from build123d import *

# Parameters (mm, degrees)
BOSS_EXTRUDE1_DEPTH                       = 12.7
BOSS_EXTRUDE1_DEPTH_BACK                  = 12.7
CUT_EXTRUDE1_DEPTH                        = 83.589067678
CUT_EXTRUDE1_DEPTH_BACK                   = 83.589067678
SKETCH5_R                                 = 3.302
BOSS_EXTRUDE_START                        = -12.7
SKETCH10_W                                = 12.7
SKETCH10_H                                = 38.1
BOSS_EXTRUDE_ARM_FB_WIDTH_DEPTH           = 44.45
BOSS_EXTRUDE_ARM_CHASSIS_FB_DEPTH         = 95.25
SKETCH15_W                                = 55.88
SKETCH15_H                                = 38.1
BOSS_EXTRUDE_ARM_CHASSIS_LR_DEPTH         = 50.8
SKETCH16_R                                = 12.7635
CUT_EXTRUDE_CHASSIS_FB_DEPTH              = 128.199614864
SKETCH17_R                                = 12.7635
SKETCH17_W                                = 12.7635
SKETCH17_H                                = 38.1
CUT_EXTRUDE_CHASSIS_LR_DEPTH              = 128.199614864
CUT_EXTRUDE_START                         = -22.107857563
CUT_EXTRUDE_CHASSIS_JOINT_CLEARANCE_DEPTH = 43.685920391
SKETCH19_W                                = 25.4
SKETCH19_H                                = 5.08
BOSS_EXTRUDE_FB_CLAMP_TOP_DEPTH           = 7.62
BOSS_EXTRUDE_START_2                      = -38.1
SKETCH19_3_W                              = 25.4
SKETCH19_3_H                              = 5.08
BOSS_EXTRUDE_FB_CLAMP_BOTTOM_DEPTH        = 7.62
SKETCH20_W                                = 5.08
SKETCH20_H                                = 25.4
BOSS_EXTRUDE_LR_CLAMP_TOP_DEPTH           = 7.62
SKETCH20_3_W                              = 5.08
SKETCH20_3_H                              = 25.4
BOSS_EXTRUDE_LR_CLAMP_BOTTOM_DEPTH        = 7.62
CHAMFER1_SIZE                             = 0.508
CHAMFER2_SIZE                             = 30.48
CHAMFER7_SIZE                             = 5.08
SKETCH26_FB_CLAMP_HOLES_R                 = 1.625000052
CUT_EXTRUDE7_FB_HOLES_DEPTH               = 136.265877047
SKETCH23_LR_CLAMP_HOLES_R                 = 1.625000052
CUT_EXTRUDE8_FB_HOLES_DEPTH               = 114.46180152
CHAMFER8_SIZE                             = 0.508


# Read off the part's stored shape, not the designer's step: Cut-Extrude Chassis Joint Clearance
with BuildPart() as part:
    # Sketch3 → Boss-Extrude1 (new, two sides: drawn at the far end of the back side and taken through both)
    with BuildSketch(Plane(origin=(0, 0, 0), x_dir=(1, 0, 0), z_dir=(0, 1, 0)).offset(-BOSS_EXTRUDE1_DEPTH_BACK)):
        with BuildLine():
            Line((8.001, 0), (10.541, 0))
            ThreePointArc((10.541, 0), (8.89018923, 5.663675172), (4.454819097, 9.553390383))
            Line((4.454819097, 9.553390383), (-5.969, 14.414097055))
            Line((-5.969, 14.414097055), (-5.969, 40.894))
            Line((-5.969, 40.894), (-18.669, 40.894))
            Line((-18.669, 40.894), (-18.669, -76.2))
            Line((-18.669, -76.2), (-5.969, -76.2))
            Line((-5.969, -76.2), (-5.969, -5.327948949))
            ThreePointArc((-5.969, -5.327948949), (-2.851142929, 7.475759828), (8.001, 0))
        make_face()
    extrude(amount=BOSS_EXTRUDE1_DEPTH + BOSS_EXTRUDE1_DEPTH_BACK)

    # Sketch5 → Cut-Extrude1 (cut, two sides: drawn at the far end of the back side and taken through both)
    with BuildSketch(Plane.ZY.offset(18.669).offset(-CUT_EXTRUDE1_DEPTH_BACK)):
        with Locations((-21.844, 0)):
            Circle(SKETCH5_R)
        with Locations((21.844, 0)):
            Circle(SKETCH5_R)
    extrude(amount=CUT_EXTRUDE1_DEPTH + CUT_EXTRUDE1_DEPTH_BACK, mode=Mode.SUBTRACT)

    # Sketch10 → Boss-Extrude Arm FB Width (add)
    with BuildSketch(Plane.XZ.offset(12.7).offset(BOSS_EXTRUDE_START)):
        with Locations((-12.319, 57.15)):
            Rectangle(SKETCH10_W, SKETCH10_H)
    extrude(amount=BOSS_EXTRUDE_ARM_FB_WIDTH_DEPTH)

    # Sketch12 → Boss-Extrude Arm Chassis FB (add)
    with BuildSketch(Plane(origin=(-5.969, 0, 0), x_dir=(0, 0, -1), z_dir=(1, 0, 0))):
        Polygon((-38.1, 0), (-76.2, 0), (-76.2, -44.45), (-38.1, -44.45), (-38.1, -12.7), align=None)
    extrude(amount=BOSS_EXTRUDE_ARM_CHASSIS_FB_DEPTH)

    # Sketch15 → Boss-Extrude Arm Chassis LR (add)
    with BuildSketch(Plane(origin=(0, 0, 0), x_dir=(1, 0, 0), z_dir=(0, 1, 0))):
        with Locations((9.271, -57.15)):
            Rectangle(SKETCH15_W, SKETCH15_H)
    extrude(amount=BOSS_EXTRUDE_ARM_CHASSIS_LR_DEPTH)

    # Sketch16 → Cut-Extrude Chassis FB (cut, through all)
    with BuildSketch(Plane(origin=(32.122028853, -6.645348837, 57.15), x_dir=(0, 0, 1), z_dir=(-1, 0, 0))):
        Circle(SKETCH16_R)
        with BuildLine():
            Line((-19.05, 0), (-12.7635, 0))
            ThreePointArc((-12.7635, 0), (-9.025157412, 9.025157392), (-2.9e-08, 12.7635))
            Line((-2.9e-08, 12.7635), (-19.05, 12.7635))
            Line((-19.05, 12.7635), (-19.05, 0))
        make_face()
        with BuildLine():
            ThreePointArc((-2.9e-08, 12.7635), (9.025157392, 9.025157412), (12.7635, 0))
            Line((12.7635, 0), (19.05, 0))
            Line((19.05, 0), (19.05, 12.7635))
            Line((19.05, 12.7635), (-2.9e-08, 12.7635))
        make_face()
    extrude(amount=-CUT_EXTRUDE_CHASSIS_FB_DEPTH, mode=Mode.SUBTRACT)

    # Sketch17 → Cut-Extrude Chassis LR (cut, through all)
    with BuildSketch(Plane(origin=(32.122028853, -6.645348837, 57.15), x_dir=(1, 0, 0), z_dir=(0, 1, 0))):
        Circle(SKETCH17_R)
        with Locations((6.38175, 0)):
            Rectangle(SKETCH17_W, SKETCH17_H)
    extrude(amount=CUT_EXTRUDE_CHASSIS_LR_DEPTH, mode=Mode.SUBTRACT)

    # Cut-Extrude Chassis Joint Clearance outl → Cut-Extrude Chassis Joint Clearance (cut)
    with BuildSketch(Plane(origin=(0, 1.051977093, 58.045037899), x_dir=(1, 0, 0), z_dir=(0, -0.11550085817456393, 0.9933073803012538)).offset(CUT_EXTRUDE_START)):
        with BuildLine():
            Line((65.60424969, 4.087995405), (49.027279167, 4.087995405))
            ThreePointArc((49.027279167, 4.087995405), (41.651365859, 10.55649777), (32.122028853, 12.8883117))
            Line((32.122028853, 12.8883117), (32.122028853, 17.444547275))
            Line((32.122028853, 17.444547275), (20.284845148, 9.156062014))
            ThreePointArc((20.284845148, 9.156062014), (17.529112657, -22.342104497), (49.027279167, -19.586372005))
            Line((49.027279167, -19.586372005), (65.60424969, 4.087995405))
        make_face()
    extrude(amount=CUT_EXTRUDE_CHASSIS_JOINT_CLEARANCE_DEPTH, mode=Mode.SUBTRACT)

    # Sketch19 → Boss-Extrude FB Clamp Top (add)
    with BuildSketch(Plane.XY.offset(76.2)):
        with Locations((76.581, -9.185348837)):
            Rectangle(SKETCH19_W, SKETCH19_H)
    extrude(amount=BOSS_EXTRUDE_FB_CLAMP_TOP_DEPTH)

    # Sketch19<3> → Boss-Extrude FB Clamp Bottom (add)
    with BuildSketch(Plane.XY.offset(76.2).offset(BOSS_EXTRUDE_START_2)):
        with Locations((76.581, -9.185348837)):
            Rectangle(SKETCH19_3_W, SKETCH19_3_H)
    extrude(amount=-BOSS_EXTRUDE_FB_CLAMP_BOTTOM_DEPTH)

    # Sketch20 → Boss-Extrude LR Clamp Top (add)
    with BuildSketch(Plane.XY.offset(76.2)):
        with Locations((29.582028853, 38.1)):
            Rectangle(SKETCH20_W, SKETCH20_H)
    extrude(amount=BOSS_EXTRUDE_LR_CLAMP_TOP_DEPTH)

    # Sketch20<3> → Boss-Extrude LR Clamp Bottom (add)
    with BuildSketch(Plane.XY.offset(76.2).offset(BOSS_EXTRUDE_START_2)):
        with Locations((29.582028853, 38.1)):
            Rectangle(SKETCH20_3_W, SKETCH20_3_H)
    extrude(amount=-BOSS_EXTRUDE_LR_CLAMP_BOTTOM_DEPTH)

    # Chamfer1
    chamfer1_edges = [part.edges().sort_by_distance(p)[0] for p in [
        (76.581, -11.725348837, 76.2),
        (76.581, -11.725348837, 38.1),
    ]]
    chamfer(chamfer1_edges, length=CHAMFER1_SIZE)

    # Chamfer2
    chamfer2_edges = [part.edges().sort_by_distance(p)[0] for p in [
        (-18.669, 50.8, 57.15),
    ]]
    chamfer(chamfer2_edges, length=CHAMFER2_SIZE)

    # Chamfer7
    chamfer7_edges = [part.edges().sort_by_distance(p)[0] for p in [
        (-12.319, 12.7, 38.1),
        (-12.319, -12.7, 38.1),
    ]]
    chamfer(chamfer7_edges, length=CHAMFER7_SIZE)

    # Sketch26 FB Clamp Holes → Cut-Extrude7 FB Holes (cut, through all)
    with BuildSketch(Plane(origin=(0, -6.645348837, 0), x_dir=(1, 0, 0), z_dir=(0, 1, 0))):
        with Locations((70.281000154, -80.01)):
            Circle(SKETCH26_FB_CLAMP_HOLES_R)
        with BuildLine():
            Line((72.264758924, -80.01), (71.612122269, -79.077938261))
            ThreePointArc((71.612122269, -79.077938261), (71.830790249, -79.52135306), (71.906000206, -80.01))
            ThreePointArc((71.906000206, -80.01), (71.830790249, -80.49864694), (71.612122269, -80.942061739))
            Line((71.612122269, -80.942061739), (72.264758924, -80.01))
        make_face()
        with BuildLine():
            Line((84.2647588, -80.01), (83.612122145, -79.077938261))
            ThreePointArc((83.612122145, -79.077938261), (83.830790125, -79.52135306), (83.906000082, -80.01))
            ThreePointArc((83.906000082, -80.01), (83.830790125, -80.49864694), (83.612122145, -80.942061739))
            Line((83.612122145, -80.942061739), (84.2647588, -80.01))
        make_face()
        with Locations((82.28100003, -80.01)):
            Circle(SKETCH26_FB_CLAMP_HOLES_R)
        with BuildLine():
            Line((84.2647588, -34.29), (83.612122145, -33.357938261))
            ThreePointArc((83.612122145, -33.357938261), (83.830790125, -33.80135306), (83.906000082, -34.29))
            ThreePointArc((83.906000082, -34.29), (83.830790125, -34.77864694), (83.612122145, -35.222061739))
            Line((83.612122145, -35.222061739), (84.2647588, -34.29))
        make_face()
        with Locations((82.28100003, -34.29)):
            Circle(SKETCH26_FB_CLAMP_HOLES_R)
        with BuildLine():
            Line((72.264758924, -34.29), (71.612122269, -33.357938261))
            ThreePointArc((71.612122269, -33.357938261), (71.830790249, -33.80135306), (71.906000206, -34.29))
            ThreePointArc((71.906000206, -34.29), (71.830790249, -34.77864694), (71.612122269, -35.222061739))
            Line((71.612122269, -35.222061739), (72.264758924, -34.29))
        make_face()
        with Locations((70.281000154, -34.29)):
            Circle(SKETCH26_FB_CLAMP_HOLES_R)
    extrude(amount=-CUT_EXTRUDE7_FB_HOLES_DEPTH, mode=Mode.SUBTRACT)

    # Sketch23 LR Clamp Holes → Cut-Extrude8 FB Holes (cut, through all)
    with BuildSketch(Plane(origin=(32.122028853, 0, 0), x_dir=(0, 0, -1), z_dir=(1, 0, 0))):
        with Locations((-80.01, 43.80000003)):
            Circle(SKETCH23_LR_CLAMP_HOLES_R)
        with Locations((-80.01, 31.800000154)):
            Circle(SKETCH23_LR_CLAMP_HOLES_R)
        with Locations(Location((-34.29, 31.800000154, 0), (0, 0, 90))):
            Circle(SKETCH23_LR_CLAMP_HOLES_R)
        with Locations(Location((-34.29, 43.80000003, 0), (0, 0, 90))):
            Circle(SKETCH23_LR_CLAMP_HOLES_R)
    extrude(amount=-CUT_EXTRUDE8_FB_HOLES_DEPTH, mode=Mode.SUBTRACT)

    # Chamfer8
    chamfer8_edges = [part.edges().sort_by_distance(p)[0] for p in [
        (27.042028853, 38.1, 76.2),
        (27.042028853, 38.1, 38.1),
    ]]
    chamfer(chamfer8_edges, length=CHAMFER8_SIZE)


solid = part.part
Verification items for the finished model (mm, model axes). A direction names the side the tool comes from. Coordinates: 2 decimals unless noted, no trailing zeros. Loops run counter-clockwise (first coordinate to the right, second up) from the corner with the lowest first, then second, coordinate; pieces in that order, holes last. Notation, with made-up numbers: (44.5, -9.75) -> (96.5, -9.75) arc R19 cw to (96.5, 0.25) -> close; hole circle Ø10 at (55, 14). An arc over 180 degrees is marked (long way). Answer as a JSON object with one key per item and string values. Group by question number.
Item 1: Sectioned sample at B-B on y = 43.8. State how many separate pieces and enclosed holes the cut face has, plus the area to 3 significant figures.
Item 2: Mould release check, pull along X, two halves, no side actions. Record for faces 1 (the cylindrical face through (80.657, -9.15, 34.232)), 2 (the flat face through (27.042, 38, 80)), 3 (the flat face through (17, 50.8, 58)): +X half, -X half, draft (parallel to the pull), parting line (faces both ways), or undercut.
Item 3: Tool access check on faces 4 (the flat face through (27.042, 38, 34)), 5 (the flat face through (-11, 12.7, -4)), 6 (the flat face through (74, -6.645, 77)), 7 (the flat face through (63.881, -9, 34)). Record the directions out of +Z, -Z, +X, -X, +Y, -Y that give a thin tool (end or side, any length) a straight path to the whole face; none if there is none.
Item 4: Sectioned sample at D-D on z = -28. Record the boundary of the cut face in (x, y).
Item 5: Depth check by flat-ended pin: pin 1 (8 mm diameter, centred on x = 75, z = 32.5, fed in from -Y); pin 2 (3 mm diameter, centred on x = 28.5, z = 80.5, fed in from -Y); pin 3 (1.5 mm diameter, centred on x = 73.5, y = -9, fed in from -Z); pin 4 (7.5 mm diameter, centred on y = 0, z = -21.844, fed in from -X). Enter the tip coordinate at first touch or a pass-through.
Item 6: Sectioned sample at A-A on x = 1. Record the boundary of the cut face in (y, z).
Item 7: Sectioned sample at C-C on y = -33. Record the boundary of the cut face in (x, z).
Item 8: Scan lines: probe 1 along X at (y, z) = (-7.9, 80.01); probe 2 along Y at (x, z) = (30.85, 80.01) (3 decimals); probe 3 along Z at (x, y) = (-14.25, 0). Record each from-to range of solid material in increasing order.
Evaluation:
{
 "1": {"separate pieces": "3", "enclosed holes": "0", "area": "829 mm²"},
 "2": {"face 1": "undercut", "face 2": "-X half", "face 3": "draft"},
 "3": {"face 4": "-Z, -X, +Y, -Y", "face 5": "-Z, +X, -X, +Y", "face 6": "+Z, -Z, +X, +Y", "face 7": "-Z, +Y, -Y"},
 "4": {"outline": "(-18.67, -12.7) -> (-5.97, -12.7) -> (-5.97, 12.7) -> (-18.67, 12.7) -> close"},
 "5": {"pin 1": "stops at y = -11.73", "pin 2": "stops at y = 25.4", "pin 3": "stops at z = 30.48", "pin 4": "stops at x = -18.67"},
 "6": {"outline": "(-44.45, 38.1) -> (39.99, 38.1) -> (39.99, 76.2) -> (-44.45, 76.2) -> close; (-12.7, -11.16) -> (12.7, -11.16) -> (12.7, -7.94) -> (-12.7, -7.94) -> close"},
 "7": {"outline": "(-18.67, 38.1) -> (89.28, 38.1) -> (89.28, 76.2) -> (-18.67, 76.2) -> close"},
 "8": {"probe 1": "x = 63.88 to 68.66, 72.26 to 80.66, 84.26 to 89.28", "probe 2": "y = 25.4 to 30.175, 33.425 to 42.175, 45.425 to 50.8", "probe 3": "z = -40.89 to -25.15, -18.54 to 18.54, 25.15 to 76.2"}
}
